from build123d import *

# Parameters (mm, degrees)
EXTRUDE_1_DEPTH     = 4
CUT_EXTRUDE_1_DEPTH = 2.55
SKETCH_3_R          = 2
CUT_EXTRUDE_2_DEPTH = 31.567792564


with BuildPart() as part:
    # 草图1 → 凸台-拉伸1 (new, symmetric)
    with BuildSketch(Plane.XY):
        with BuildLine():
            Line((0, 0), (15, 0))
            Line((15, 0), (23.511091256, -11.091870075))
            ThreePointArc((23.511091256, -11.091870075), (23.706523759, -11.849971903), (23.295917311, -12.516541172))
            ThreePointArc((23.295917311, -12.516541172), (7.5, -17.545906941), (-8.295917311, -12.516541172))
            ThreePointArc((-8.295917311, -12.516541172), (-8.706523759, -11.849971903), (-8.511091256, -11.091870075))
            Line((-8.511091256, -11.091870075), (0, 0))
        make_face()
    extrude(amount=EXTRUDE_1_DEPTH, both=True)

    # 草图2 → 切除-拉伸1 (cut, symmetric)
    with BuildSketch(Plane.XY):
        with BuildLine():
            Line((1.45, 0), (1.45, -6))
            ThreePointArc((1.45, -6), (7.5, -12.05), (13.55, -6))
            Line((13.55, -6), (13.55, 0))
            Line((13.55, 0), (1.45, 0))
        make_face()
    extrude(amount=CUT_EXTRUDE_1_DEPTH, both=True, mode=Mode.SUBTRACT)

    # 草图3 → 切除-拉伸2 (cut, through all)
    with BuildSketch(Plane.XY.offset(4)):
        with Locations((7.5, -6)):
            Circle(SKETCH_3_R)
    extrude(amount=-CUT_EXTRUDE_2_DEPTH, mode=Mode.SUBTRACT)


solid = part.part
The model under review builds one solid part; all positions refer to its coordinate system, in mm. A direction names the side the tool comes from. Coordinates: 2 decimals unless noted, no trailing zeros. Write each loop counter-clockwise with the first axis right and the second up, starting at its lowest first coordinate (ties: lowest second). Pieces come first, ordered by that corner, then holes. Notation, with made-up numbers: M 11.25,30 L 43.25,30 A7 ccw 43.25,37 Z; hole C -34.5,-7 d1. An arc over 180 degrees is marked long. Put each result on its own line as item: value.
1) For faces 5 (the cylindrical face through (7.736, -17.545, 0.056)), 6 (the flat face through (13.55, -3, 0)), list the 3-axis set-ups (+Z, -Z, +X, -X, +Y, -Y) from which the entire face can be reached by the end or side of a thin tool; tool diameter is ignored.
Computed:
face 5: +Z, -Z, -Y
face 6: +Y
2) Draft analysis for pull direction Y (two halves, no side actions). For faces 1 (the flat face through (7, -3, 2.55)), 2 (the cylindrical face through (5.502, -5.912, -3.265)), 3 (the cylindrical face through (5.502, -5.912, 3.285)), 4 (the flat face through (19.196, -5.468, 0.056)), state which applies: released by +Y, released by -Y, zero draft, split by the parting line, or undercut.
Computed:
face 1: zero draft
face 2: undercut
face 3: undercut
face 4: released by +Y
3) Clearance check with flat-ended pins moving along their axes: pin 1 Ø1.5 at (y, z) = (-4, 1) entering from +X; pin 2 Ø2 at (x, z) = (1.5, 0.5) entering from -Y; pin 3 Ø1.5 at (x, z) = (0.5, -1) entering from -Y. State where each tip first meets the part, or that it passes through.
Computed:
pin 1: stops at x = 18.64
pin 2: stops at y = -17.08
pin 3: stops at y = -16.82
4) Add section A-A on z = 0.75. Give the boundary of the cut face in (x, y).
Computed:
outline: M -8.51,-11.09 A1 ccw -8.3,-12.52 A27.32 ccw 23.3,-12.52 A1 ccw 23.51,-11.09 L 15,0 L 13.55,0 L 13.55,-6 A6.05 cw 1.45,-6 L 1.45,0 L 0,0 Z
5) Add section B-B on x = 7.5. Give the boundary of the cut face in (y, z).
Computed:
outline: M -17.55,-4 L -8,-4 L -8,-2.55 L -12.05,-2.55 L -12.05,2.55 L -8,2.55 L -8,4 L -17.55,4 Z; M -4,-4 L 0,-4 L 0,-2.55 L -4,-2.55 Z; M -4,2.55 L 0,2.55 L 0,4 L -4,4 Z
6) Wall thickness on probe 1 along Y at (x, z) = (7.5, 3.4); probe 2 along Z at (x, y) = (3, -10); probe 3 along X at (y, z) = (-5.5, -0.5): over which ranges is each line inside the solid? List them lowest first. Write a range as [from, to].
Computed:
probe 1: y = [-17.55, -8], [-4, 0]
probe 2: z = [-4, -2.55], [2.55, 4]
probe 3: x = [-4.22, 1.45], [13.55, 19.22]
7) Add section D-D on x = 4. Give the boundary of the cut face in (y, z), then the cut area to 3 significant figures.
Computed:
outline: M -17.32,-4 L 0,-4 L 0,-2.55 L -10.93,-2.55 L -10.93,2.55 L 0,2.55 L 0,4 L -17.32,4 Z
area: 82.8 mm2
8) Add section C-C on y = -10.25. Give the boundary of the cut face in (x, z).
Computed:
outline: M -7.87,-4 L 22.87,-4 L 22.87,4 L -7.87,4 Z; hole M 3.19,-2.55 L 11.81,-2.55 L 11.81,2.55 L 3.19,2.55 Z
